Part print with two shaded views. Sizes in mm from the minimum x, y, z corner. A direction names the side the tool comes from. Coordinates: 2 decimals unless noted, no trailing zeros. Write each loop counter-clockwise with the first axis right and the second up, starting at its lowest first coordinate (ties: lowest second). Pieces come first, ordered by that corner, then holes. Notation, with made-up numbers: (38, -30.75) - (83, -30.75) arc R19 cw to (83, -22.75) - close; hole circle Ø10 at (53.5, 19.25). An arc over 180 degrees is marked (long way). One line per question, with ' | ' between items. Start each with the question number.
1. Which spindle directions (+Z, -Z, +X, -X, +Y, -Y) get a long thin tool onto all of the face, cutting with end or side? Do the marked faces 5, 6 and 7. Say none if no direction does.
2. Band-saw the part on D-D, the plane z = 28. Write the cut outline in (x, y).
3. Probe line 1 (Y direction, x = 27, z = 16); line 2 (X direction, y = 99, z = 3); line 3 (Y direction, x = 5, z = 17). List the from-to ranges inside material, lowest first.
4. Two-plate mould, pull along Y, no slides. Class the marked faces 1, 2, 3 and 4: +Y half, -Y half, draft (parallel to the pull), parting line (faces both ways), or undercut.
5. Flat gauge pins, fed straight in: P1, Ø6, axis at y = 85.5, z = 26.5, coming from the +X side; P2, Ø1, axis at y = 95.5, z = 28, coming from the +X side; P3, Ø2, axis at y = 90.5, z = 14.5, coming from the +X side. Where does each tip first touch, or does it go through?
6. Band-saw the part on C-C, the plane x = 2.5. Write the cut outline in (y, z), then the cut area to 3 significant figures.
7. Band-saw the part on B-B, the plane x = 16. Write the cut outline in (y, z), then the cut area to 3 significant figures.
8. Band-saw the part on A-A, the plane z = 16. Write the cut outline in (x, y).
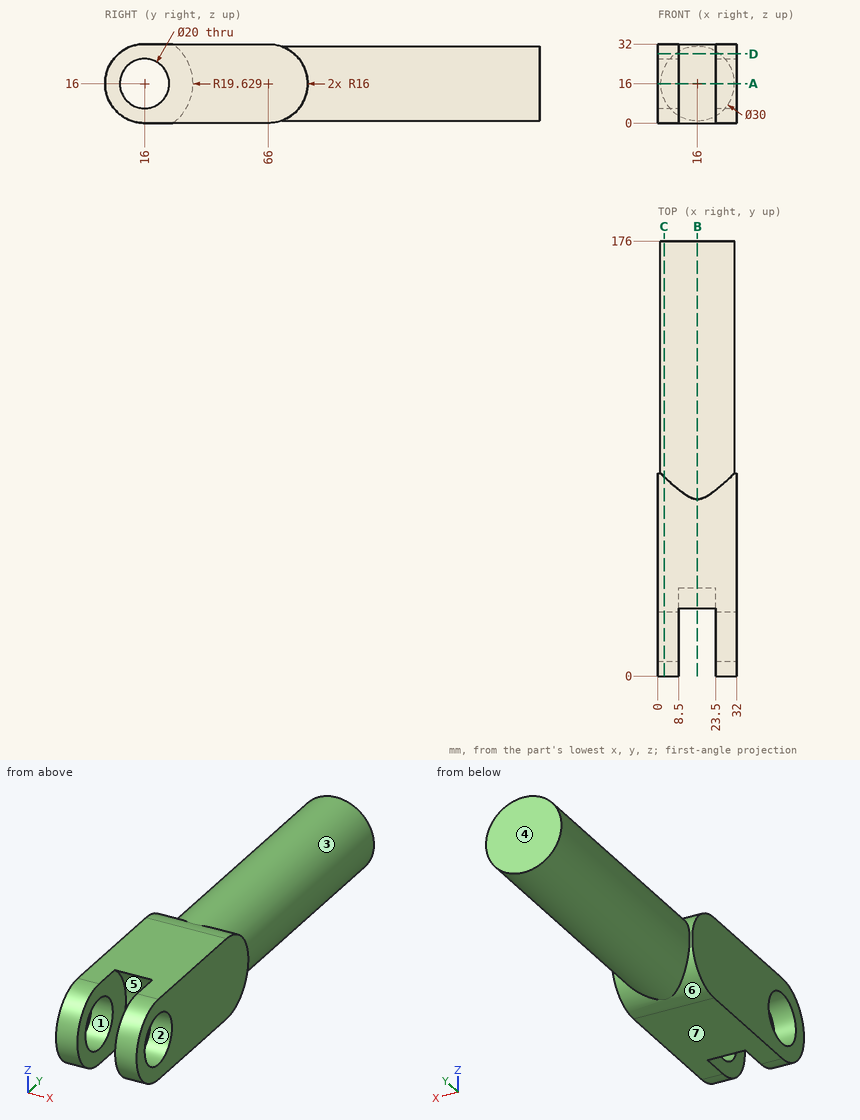
Filled in:
1) face 5: -Y | face 6: +Y | face 7: -Z, +X, -X, +Y, -Y
2) outline: (0, 5.42) - (8.5, 5.42) - (8.5, 31.53) - (23.5, 31.53) - (23.5, 5.42) - (32, 5.42) - (32, 76.58) - (25, 76.58) - (25, 176) - (7, 176) - (7, 76.58) - (0, 76.58) - close
3) line 1: y = 0 to 6, 26 to 176 | line 2: x = 8.52 to 23.48 | line 3: y = 0.03 to 6.05, 25.95 to 176
4) face 1: undercut | face 2: undercut | face 3: draft | face 4: +Y half
5) P1: stops at x = 28.99 | P2: stops at x = 25.63 | P3: stops at x = 30.99
6) outline: (16, 0) - (66, 0) arc R16 ccw to (80.6, 9.46) - (176, 9.46) - (176, 22.54) - (80.6, 22.54) arc R16 ccw to (66, 32) - (16, 32) arc R16 ccw to start; hole circle Ø20 at (16, 16) | area: 3,330 mm²
7) outline: (27.37, 0) - (66, 0) arc R16 ccw to (71.57, 1) - (176, 1) - (176, 31) - (71.57, 31) arc R16 ccw to (66, 32) - (27.37, 32) arc R19.63 cw to start | area: 4,360 mm²
8) outline: (0, 0) - (8.5, 0) - (8.5, 6) - (0, 6) - close; (0, 26) - (8.5, 26) - (8.5, 35.63) - (23.5, 35.63) - (23.5, 26) - (32, 26) - (32, 82) - (31, 82) - (31, 176) - (1, 176) - (1, 82) - (0, 82) - close; (23.5, 0) - (32, 0) - (32, 6) - (23.5, 6) - close
